Geometry check sheet. Reference: drawing and pictorial views, mm from the part's lowest x, y, z. Give positions to 0.01 mm unless a question says otherwise; leave off trailing zeros. Order: outer loops, then holes, each group sorted by start corner. A loop starts at its lowest first (then second) coordinate and runs counter-clockwise, first axis right, second up. Notation, with made-up numbers: (51, -14) -> (103, -14) arc R17 ccw to (103, -5) -> close; hole circle Ø4 at (19, 54). An arc over 180 degrees is marked (long way). Write each question's results on one line, items separated by ' | '.
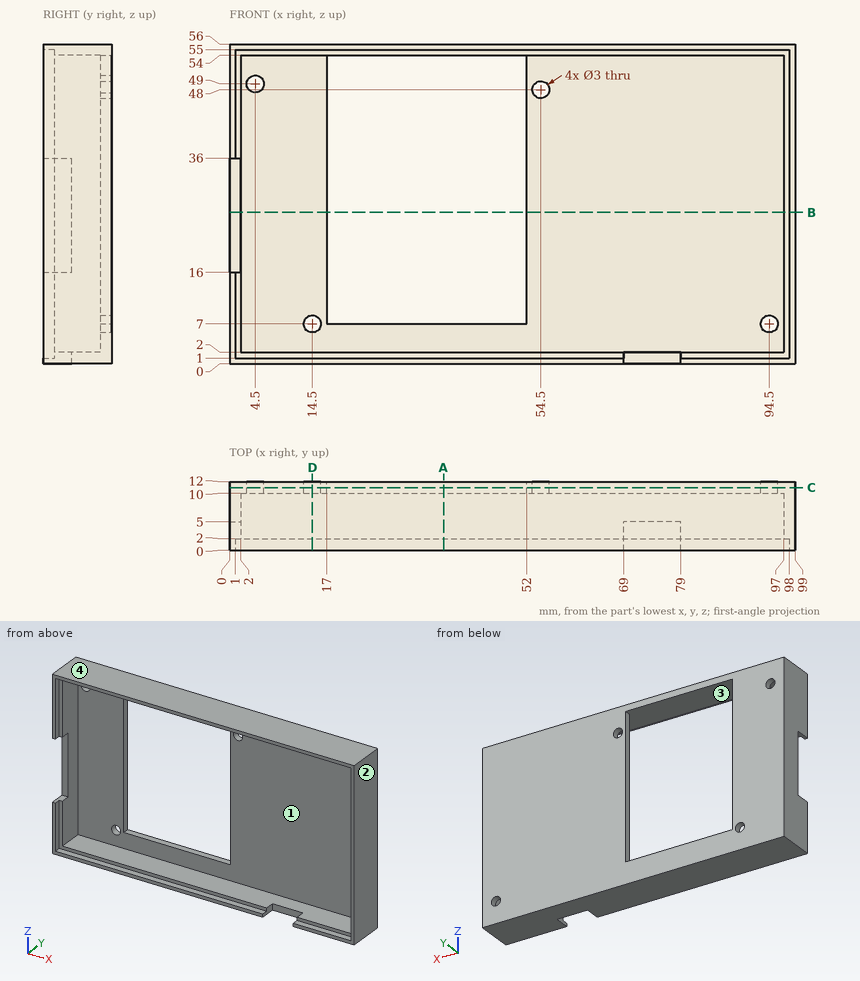
1. Gauge pin test, flat ends, axial feed: pin 1 Ø5 at (x, y) = (29, 10) entering from -Z; pin 2 Ø2.5 at (x, z) = (94.5, 7) entering from -Y; pin 3 Ø0.6 at (x, z) = (74.5, 1.5) entering from -Y; pin 4 Ø7.5 at (x, z) = (21, 7.5) entering from -Y. Record the tip position at first contact, or that the pin passes through.
Verdict:
pin 1: stops at z = 0 | pin 2: passes through | pin 3: stops at y = 5 | pin 4: stops at y = 10
2. Section check D-D on x = 14.5. Record the cut outline in (y, z).
Verdict:
outline: (0, 0) -> (12, 0) -> (12, 5.5) -> (10, 5.5) -> (10, 2) -> (2, 2) -> (2, 1) -> (0, 1) -> close; (0, 55) -> (2, 55) -> (2, 54) -> (10, 54) -> (10, 8.5) -> (12, 8.5) -> (12, 56) -> (0, 56) -> close
3. Mould release check, pull along X, two halves, no side actions. Record for the marked faces 1, 2, 3 and 4: +X half, -X half, draft (parallel to the pull), parting line (faces both ways), or undercut.
Verdict:
face 1: undercut | face 2: +X half | face 3: undercut | face 4: draft
4. Material ranges on probe 1 along Z at (x, y) = (88.5, 4.25); probe 2 along Z at (x, y) = (94.5, 10.65); probe 3 along X at (y, z) = (11.5, 49), recorded low to high. Write a range as from..to.
Verdict:
probe 1: z = 0..2, 54..56 | probe 2: z = 0..5.5, 8.5..56 | probe 3: x = 0..3, 6..17, 52..53.38, 55.62..99
5. Section check C-C on y = 11. Record the cut outline in (x, z).
Verdict:
outline: (0, 0) -> (99, 0) -> (99, 56) -> (0, 56) -> close; hole circle Ø3 at (4.5, 49); hole circle Ø3 at (14.5, 7); hole (17, 7) -> (52, 7) -> (52, 54) -> (17, 54) -> close; hole circle Ø3 at (54.5, 48); hole circle Ø3 at (94.5, 7)
6. Section check B-B on z = 26.5. Record the cut outline in (x, y), then the cut area to 3 significant figures.
Verdict:
outline: (0, 5) -> (2, 5) -> (2, 10) -> (17, 10) -> (17, 12) -> (0, 12) -> close; (52, 10) -> (97, 10) -> (97, 2) -> (98, 2) -> (98, 0) -> (99, 0) -> (99, 12) -> (52, 12) -> close | area: 156 mm^2
7. Section check A-A on x = 37.5. Record the cut outline in (y, z).
Verdict:
outline: (0, 0) -> (12, 0) -> (12, 7) -> (10, 7) -> (10, 2) -> (2, 2) -> (2, 1) -> (0, 1) -> close; (0, 55) -> (2, 55) -> (2, 54) -> (12, 54) -> (12, 56) -> (0, 56) -> close
